Autodesk Inventor part; units mm, degrees
ref_plane "YZ Plane" through (0, 0, 0) normal (1, 0, 0) x (0, 1, 0)
ref_plane "XZ Plane" through (0, 0, 0) normal (0, 1, 0) x (-1, 0, 0)
ref_plane "XY Plane" through (0, 0, 0) normal (0, 0, 1) x (1, 0, 0)
sketch "Sketch1" plane through (0, 0, 0) normal (0, 1, 0) x (-1, 0, 0)
  circle A0 centre (0, 0) radius 335
  dimension "d0" = 670
extrude "Extrusion1" add sketch "Sketch1" along normal blind 8
sketch "Sketch2" plane through (0, 8, 0) normal (0, 1, 0) x (1, 0, 0)
  circle A0 centre (0, 0) radius 310 construction
  line L0 (0, 0) -> (-310, 0)
  line L1 (0, 0) -> (-306.1834, 48.4947) construction
  point P0 (-306.1834, -48.4947)
  point P1 (-306.1834, -48.4947)
  point P2 (-276.212, -140.7371)
  point P3 (-276.212, -140.7371)
  point P4 (-219.2031, -219.2031)
  point P5 (-219.2031, -219.2031)
  point P6 (-140.7371, -276.212)
  point P7 (-140.7371, -276.212)
  point P8 (-48.4947, -306.1834)
  point P9 (-48.4947, -306.1834)
  point P10 (48.4947, -306.1834)
  point P11 (48.4947, -306.1834)
  point P12 (140.7371, -276.212)
  point P13 (140.7371, -276.212)
  point P14 (219.2031, -219.2031)
  point P15 (219.2031, -219.2031)
  point P16 (276.212, -140.7371)
  point P17 (276.212, -140.7371)
  point P18 (306.1834, -48.4947)
  point P19 (306.1834, -48.4947)
  point P20 (306.1834, 48.4947)
  point P21 (306.1834, 48.4947)
  point P22 (276.212, 140.7371)
  point P23 (276.212, 140.7371)
  point P24 (219.2031, 219.2031)
  point P25 (219.2031, 219.2031)
  point P26 (140.7371, 276.212)
  point P27 (140.7371, 276.212)
  point P28 (48.4947, 306.1834)
  point P29 (48.4947, 306.1834)
  point P30 (-48.4947, 306.1834)
  point P31 (-48.4947, 306.1834)
  point P32 (-140.7371, 276.212)
  point P33 (-140.7371, 276.212)
  point P34 (-219.2031, 219.2031)
  point P35 (-219.2031, 219.2031)
  point P36 (-276.212, 140.7371)
  point P37 (-276.212, 140.7371)
  dimension "d4" = 620
  dimension "d11" = 9
  dimension "d24" = 360
hole "Hole2" at (-306.1834, 8, -48.4947) at (-306.1834, 8, 48.4947) at (-276.212, 8, 140.7371) at (-219.2031, 8, 219.2031) at (-140.7371, 8, 276.212) at (-48.4947, 8, 306.1834) at (48.4947, 8, 306.1834) at (140.7371, 8, 276.212) at (219.2031, 8, 219.2031) at (276.212, 8, 140.7371) at (306.1834, 8, 48.4947) at (306.1834, 8, -48.4947) at (276.212, 8, -140.7371) at (219.2031, 8, -219.2031) at (140.7371, 8, -276.212) at (48.4947, 8, -306.1834) at (-48.4947, 8, -306.1834) at (-140.7371, 8, -276.212) at (-219.2031, 8, -219.2031) at (-276.212, 8, -140.7371) direction (0, -1, 0) diameter 26 end through all
equation "\"d1\" = Thickness"
equation "\"BendRadius\" = Thickness"
equation "\"BendReliefWidth\" = Thickness"
equation "\"BendReliefDepth\" = 0.5 * Thickness"
equation "\"CornerReliefSize\" = 4 * Thickness"
equation "\"MinimumRemnant\" = 2 * Thickness"
equation "\"TransitionRadius\" = BendRadius"
equation "\"JacobiRadiusSize\" = BendRadius"
equation "\"GapSize\" = Thickness"
equation "\"d5\" = Thickness"
properties part number "PRS 1621 charging hatch D1200 940"
Part model, mm, in its own coordinate system. Give positions to 0.01 mm unless a question says otherwise; leave off trailing zeros. Order: outer loops, then holes, each group sorted by start corner. A loop starts at its lowest first (then second) coordinate and runs counter-clockwise, first axis right, second up. Notation, with made-up numbers: (39.5, 88.25) -> (71.5, 88.25) arc R28 ccw to (71.5, 120.25) -> close; hole circle Ø10 at (59.5, 14). An arc over 180 degrees is marked (long way). Use one line per item in the form item = value.
(1) Flat gauge pins, fed straight in: P1, Ø1, axis at y = 1.5, z = -164, coming from the -X side; P2, Ø21, axis at x = -219.2, z = 219.2, coming from the +Y side; P3, Ø1.5, axis at x = 83, y = 1, coming from the -Z side. Where does each tip first touch, or does it go through?
Solution:
P1 = -292.39
P2 = through
P3 = -324.75
(2) Pull direction Z, two halves, no side cores. Call faces 1 (the face through (-268.3, 3.94, 130.42)), 2 (the face through (5, 8, 5)), 3 (the face through (265.845, 3.944, 203.842)): +Z half, -Z half, draft (parallel to the pull), parting line (faces both ways), or undercut.
Solution:
face_1 = undercut
face_2 = draft
face_3 = parting line
(3) Saw through at B-B (x = 80.5). Write the cut outline in (y, z), then the cut area to 3 significant figures.
Solution:
outline = (0, -325.18) -> (8, -325.18) -> (8, 325.18) -> (0, 325.18) -> close
area = 5,200 mm²
(4) Drill centre lines: line 1 (X direction, y = 5.5, z = -283.5); line 2 (X direction, y = 6.5, z = 228); line 3 (Z direction, x = -46, y = 6). Where is each one in solid material? Low to high. Write a range as from..to.
Solution:
line_1 = -178.47..-151.5, -129.97..129.97, 151.5..178.47
line_2 = -245.44..-228.77, -209.63..209.63, 228.77..245.44
line_3 = -331.83..-318.94, -293.43..293.43, 318.94..331.83
(5) Saw through at C-C (z = -240). Write the cut outline in (x, y).
Solution:
outline = (-233.72, 0) -> (233.72, 0) -> (233.72, 8) -> (-233.72, 8) -> close
(6) Saw through at A-A (y = 1.5). Count the separate pieces of the cut face and the enclosed holes in it, then the cut area to 3 significant figures.
Solution:
separate_pieces = 1
enclosed_holes = 20
area = 342,000 mm²
